For this review, take the finished solid that the model builds, in its own axes (mm). A direction names the side the tool comes from. Round coordinates to 2 decimals unless told otherwise and drop trailing zeros. Order: outer loops, then holes, each group sorted by start corner. A loop starts at its lowest first (then second) coordinate and runs counter-clockwise, first axis right, second up.
from build123d import *

# Parameters (mm, degrees)
F0_R     = 11.5
F0_W     = 20
F0_H     = 20
F0_R_2   = 3
F1_DEPTH = 10.5
F0_R_3   = 10.5
F2_DEPTH = 2
F3_R     = 3


with BuildPart() as f1:
    # F0 (on Top) → F1 (new body)
    with BuildSketch(Plane.XY):
        Polygon((25, 17.5), (-25, 17.5), (-25, 10), (-25, -10), (-25, -17.5), (25, -17.5), (25, -10), (25, 10), align=None)
        Circle(F0_R, mode=Mode.SUBTRACT)
        with Locations((-35, 0)):
            Rectangle(F0_W, F0_H)
        with Locations((-35, 0)):
            Circle(F0_R_2, mode=Mode.SUBTRACT)
        with Locations((35, 0)):
            Rectangle(F0_W, F0_H)
        with Locations((35, 0)):
            Circle(F0_R_2, mode=Mode.SUBTRACT)
    extrude(amount=F1_DEPTH)

    # F0 (on Top) → F2 (join)
    with BuildSketch(Plane.XY):
        Circle(F0_R)
        Circle(F0_R_3, mode=Mode.SUBTRACT)
    extrude(amount=F2_DEPTH)

    # F3
    f3_edges = [f1.edges().sort_by_distance(p)[0] for p in [
        (-25, -10, 5.25),
        (-25, 10, 5.25),
        (25, 10, 5.25),
        (25, -10, 5.25),
        (25, 17.5, 5.25),
        (25, -17.5, 5.25),
        (-25, -17.5, 5.25),
        (-25, 17.5, 5.25),
        (-45, 10, 5.25),
        (-45, -10, 5.25),
        (45, -10, 5.25),
        (45, 10, 5.25),
    ]]
    fillet(f3_edges, radius=F3_R)


solid = f1.part
(1) Add section A-A on x = 0. Give the boundary of the cut face in (y, z), plus the area to 3 significant figures.
(2) Add section B-B on z = 5.25. Give the boundary of the cut face in (x, y), plus the area to 3 significant figures.
(3) Clearance check with flat-ended pins moving along their axes: P1, Ø1.2, axis at y = 13.5, z = 3, coming from the -X side; P2, Ø1, axis at y = -12.5, z = 3, coming from the -X side; P3, Ø3, axis at x = -33, z = 6.5, coming from the +Y side; P4, Ø8, axis at x = 7, y = 5.5, coming from the -Z side. State where each tip first meets the part, or that it passes through.
(4) Tool access review of faces 1 (the face through (35, 10, 5)), 2 (the face through (35, -10, 5)), 3 (the face through (3.4, -10.2, 2)), 4 (the face through (-1, 12, 10.5)): name each direction out of +Z, -Z, +X, -X, +Y, -Y from which nothing blocks a thin tool from reaching the whole face with its end or side.
(5) Draft analysis for pull direction X (two halves, no side actions). For faces 5 (the face through (-25, -14, 5)), 6 (the face through (32, 0, 5)), 7 (the face through (25.86, 10.9, 5.32)), state which applies: pulls with the +X half, pulls with the -X half, needs draft (parallel to the pull), parting line crosses it, or undercut.
(6) Add section C-C on y = 0. Give the boundary of the cut face in (x, z), plus the area to 4 significant figures.
(7) Add section D-D on y = 8. Give the boundary of the cut face in (x, z).
(8) Wall thickness on L1, parallel to Y at x = 35, z = 3.5; L2, parallel to X at y = 2, z = 5; L3, parallel to Y at x = 0, z = 0.9: over which ranges is each line inside the solid? List them lowest first.
Here are the results:
1. outline: (-17.5, 0) - (-10.5, 0) - (-10.5, 2) - (-11.5, 2) - (-11.5, 10.5) - (-17.5, 10.5) - close; (10.5, 0) - (17.5, 0) - (17.5, 10.5) - (11.5, 10.5) - (11.5, 2) - (10.5, 2) - close
1. area: 130 mm2
2. outline: (-45, -7) arc R3 ccw to (-42, -10) - (-28, -10) arc R3 cw to (-25, -13) - (-25, -14.5) arc R3 ccw to (-22, -17.5) - (22, -17.5) arc R3 ccw to (25, -14.5) - (25, -13) arc R3 cw to (28, -10) - (42, -10) arc R3 ccw to (45, -7) - (45, 7) arc R3 ccw to (42, 10) - (28, 10) arc R3 cw to (25, 13) - (25, 14.5) arc R3 ccw to (22, 17.5) - (-22, 17.5) arc R3 ccw to (-25, 14.5) - (-25, 13) arc R3 cw to (-28, 10) - (-42, 10) arc R3 ccw to (-45, 7) - close; hole circle Ø6 at (-35, 0); hole circle Ø23 at (0, 0); hole circle Ø6 at (35, 0)
2. area: 2,070 mm2
3. P1: stops at x = -25
3. P2: stops at x = -25.17
3. P3: stops at y = 10
3. P4: stops at z = 0
4. face 1: +Z, -Z, +X, +Y
4. face 2: +Z, -Z, +X, -Y
4. face 3: +Z
4. face 4: +Z, +X, -X, +Y, -Y
5. face 5: pulls with the -X half
5. face 6: undercut
5. face 7: pulls with the +X half
6. outline: (-45, 0) - (-38, 0) - (-38, 10.5) - (-45, 10.5) - close; (-32, 0) - (-10.5, 0) - (-10.5, 2) - (-11.5, 2) - (-11.5, 10.5) - (-32, 10.5) - close; (10.5, 0) - (32, 0) - (32, 10.5) - (11.5, 10.5) - (11.5, 2) - (10.5, 2) - close; (38, 0) - (45, 0) - (45, 10.5) - (38, 10.5) - close
6. area: 581.5 mm2
7. outline: (-44.83, 0) - (-6.8, 0) - (-6.8, 2) - (-8.26, 2) - (-8.26, 10.5) - (-44.83, 10.5) - close; (6.8, 0) - (44.83, 0) - (44.83, 10.5) - (8.26, 10.5) - (8.26, 2) - (6.8, 2) - close
8. L1: y = -10 to -3, 3 to 10
8. L2: x = -45 to -37.24, -32.76 to -11.32, 11.32 to 32.76, 37.24 to 45
8. L3: y = -17.5 to -10.5, 10.5 to 17.5
